```python
from build123d import *

# Parameters (mm, degrees)
BOSS_EXTRUDE1_DEPTH = 12.7
SKETCH2_W           = 190.5
SKETCH2_H           = 114.3
CUT_EXTRUDE1_DEPTH  = 6.35


with BuildPart() as part:
    # Sketch1 → Boss-Extrude1 (new body)
    with BuildSketch(Plane(origin=(0, 0, 0), x_dir=(1, 0, 0), z_dir=(0, 1, 0))):
        Polygon((-101.6, 44.45), (-50.8, 44.45), (-50.8, 63.5), (101.6, 63.5), (101.6, -63.5), (-50.8, -63.5), (-50.8, -44.45), (-101.6, -44.45), align=None)
    extrude(amount=BOSS_EXTRUDE1_DEPTH)

    # Sketch2 → Cut-Extrude1 (cut)
    with BuildSketch(Plane(origin=(0, 12.7, 0), x_dir=(1, 0, 0), z_dir=(0, 1, 0))):
        Rectangle(SKETCH2_W, SKETCH2_H)
    extrude(amount=-CUT_EXTRUDE1_DEPTH, mode=Mode.SUBTRACT)


solid = part.part
```
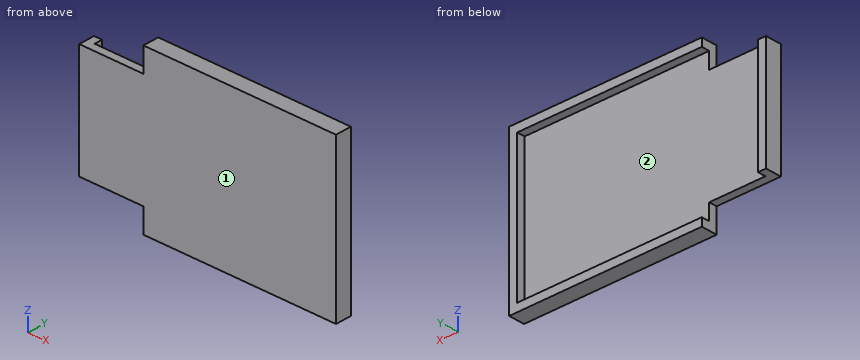
CAD build for the part. Positions are in the model's coordinates, mm. Face numbers are marked on the shaded views. Round coordinates to 2 decimals unless told otherwise and drop trailing zeros. Loops run counter-clockwise (first coordinate to the right, second up) from the corner with the lowest first, then second, coordinate; pieces in that order, holes last. Notation, with made-up numbers: (2.5, 71) - (51.5, 71) arc R18 cw to (51.5, 88) - close; hole circle Ø1 at (-12, 28.5). An arc over 180 degrees is marked (long way). Return JSON: item names as keys, results as strings. Group by question number.
Q1. Flat gauge pins, fed straight in: pin 1 Ø6.5 at (y, z) = (9, -53.5) entering from -X; pin 2 Ø6 at (x, z) = (-38.5, 1.5) entering from +Y; pin 3 Ø4 at (x, y) = (-55.5, 5.5) entering from -Z. Where does each tip first touch, or does it go through?
Q2. Band-saw the part on A-A on y = 9.75. Give the cut face in (x, z), plus the area to 3 significant figures.
Q3. Band-saw the part on B-B on z = 41.5. Give the cut face in (x, y), plus the area to 3 significant figures.
Q4. Band-saw the part on C-C on x = 31.5. Give the cut face in (y, z), plus the area to 3 significant figures.
Q5. Two-plate mould, pull along X, no slides. Class the marked faces 1 and 2: +X half, -X half, draft (parallel to the pull), parting line (faces both ways), or undercut.
Q6. Band-saw the part on D-D on z = -54. Give the cut face in (x, y), plus the area to 3 significant figures.
Q7. Drill centre lines: line 1 along Z through (x, y) = (-13, 11); line 2 along X through (y, z) = (8.25, -27.5); line 3 along Y through (x, z) = (-86.5, 16). Where is each one in solid material? Low to high. Write a range as [from, to].
Solutions:
{
 "1": {"pin 1": "stops at x = -50.8", "pin 2": "stops at y = 6.35", "pin 3": "stops at z = -44.45"},
 "2": {"outline": "(-101.6, -44.45) - (-95.25, -44.45) - (-95.25, 44.45) - (-101.6, 44.45) - close; (-50.8, -63.5) - (101.6, -63.5) - (101.6, 63.5) - (-50.8, 63.5) - (-50.8, 57.15) - (95.25, 57.15) - (95.25, -57.15) - (-50.8, -57.15) - close", "area": "3,230 mm^2"},
 "3": {"outline": "(-101.6, 0) - (101.6, 0) - (101.6, 12.7) - (95.25, 12.7) - (95.25, 6.35) - (-95.25, 6.35) - (-95.25, 12.7) - (-101.6, 12.7) - close", "area": "1,370 mm^2"},
 "4": {"outline": "(0, -63.5) - (12.7, -63.5) - (12.7, -57.15) - (6.35, -57.15) - (6.35, 57.15) - (12.7, 57.15) - (12.7, 63.5) - (0, 63.5) - close", "area": "887 mm^2"},
 "5": {"face 1": "draft", "face 2": "undercut"},
 "6": {"outline": "(-50.8, 0) - (101.6, 0) - (101.6, 12.7) - (95.25, 12.7) - (95.25, 6.35) - (-50.8, 6.35) - close", "area": "1,010 mm^2"},
 "7": {"line 1": "z = [-63.5, -57.15], [57.15, 63.5]", "line 2": "x = [-101.6, -95.25], [95.25, 101.6]", "line 3": "y = [0, 6.35]"}
}
